from build123d import *

# Parameters (mm, degrees)
BOSS_EXTRUDE1_DEPTH = 4
SKETCH2_R           = 2.5
CUT_EXTRUDE1_DEPTH  = 4
LPATTERN1_COUNT     = 3
LPATTERN1_PITCH     = 20
SKETCH3_R           = 2.5
CUT_EXTRUDE2_DEPTH  = 4
FILLET1_R           = 0.1


with BuildPart() as part:
    # Sketch1 → Boss-Extrude1 (new body)
    with BuildSketch(Plane.XY):
        Polygon((20, 60), (40, 60), (60, 20), (60, 0), (0, 0), (0, 20), align=None)
    extrude(amount=-BOSS_EXTRUDE1_DEPTH)

    # Sketch2 → Cut-Extrude1 (cut)
    with BuildSketch(Plane.XY):
        with Locations((30, 10)):
            Circle(SKETCH2_R)
    cut_extrude1 = extrude(amount=-CUT_EXTRUDE1_DEPTH, mode=Mode.SUBTRACT)

    # LPattern1: Cut-Extrude1 ×3
    with Locations(*[(0, i * LPATTERN1_PITCH, 0) for i in range(1, LPATTERN1_COUNT)]):
        add(cut_extrude1, mode=Mode.SUBTRACT)

    # Sketch3 → Cut-Extrude2 (cut)
    with BuildSketch(Plane.XY):
        with Locations((10, 10)):
            Circle(SKETCH3_R)
        with Locations((50, 10)):
            Circle(SKETCH3_R)
    extrude(amount=-CUT_EXTRUDE2_DEPTH, mode=Mode.SUBTRACT)

    # Fillet1
    fillet1_edges = [part.edges().sort_by_distance(p)[0] for p in [
        (0, 0, -2),
        (0, 20, -2),
        (20, 60, -2),
        (40, 60, -2),
        (60, 20, -2),
        (60, 0, -2),
    ]]
    fillet(fillet1_edges, radius=FILLET1_R)


solid = part.part
Work out the finished part from the listing and answer in its coordinate system (mm). Round coordinates to 2 decimals unless told otherwise and drop trailing zeros. Write each loop counter-clockwise with the first axis right and the second up, starting at its lowest first coordinate (ties: lowest second). Pieces come first, ordered by that corner, then holes. Notation, with made-up numbers: (74.5, -8.75) -> (92.5, -8.75) arc R25 cw to (92.5, 16.25) -> close; hole circle Ø2 at (-15, 47). An arc over 180 degrees is marked (long way). Answer as CSV lines item,"result". Start each with the question number.
(1) The part is cut by section C-C, the plane x = 30. Give the vertices of the cut face in (y, z).
(2) Find the intervals of material crossed by probe 1 along Y at (x, z) = (30, -2.7); probe 2 along Y at (x, z) = (29, -1.85); probe 3 along Y at (x, z) = (10, -2.95), in increasing order.
(3) The part is cut by section A-A, the plane y = 31.5. Give the vertices of the cut face in (x, z).
(4) Each of these flat-tipped pins is pushed along its axis until it touches: pin 1 (8 mm diameter, centred on x = 15, y = 53, fed in from +Z); pin 2 (1 mm diameter, centred on y = 49.5, z = -3.5, fed in from +X). Where does it stop, or does it pass through?
(5) The mould has two halves that part along Y. Classify faces 1 (the cylindrical face through (28.16, 51.69, -1.97)), 2 (the flat face through (30, 0, -2)), 3 (the flat face through (10, 40, -2)), 4 (the flat face through (0, 10, -2)): +Y half, -Y half, draft (parallel to the pull), parting line (faces both ways), or undercut.
(6) The part is cut by section B-B, the plane z = -2.55. Give the vertices of the cut face in (x, y).
Output values:
1,outline,"(0, -4) -> (7.5, -4) -> (7.5, 0) -> (0, 0) -> close; (12.5, -4) -> (27.5, -4) -> (27.5, 0) -> (12.5, 0) -> close; (32.5, -4) -> (47.5, -4) -> (47.5, 0) -> (32.5, 0) -> close; (52.5, -4) -> (60, -4) -> (60, 0) -> (52.5, 0) -> close"
2,probe 1,"y = 0 to 7.5, 12.5 to 27.5, 32.5 to 47.5, 52.5 to 60"
2,probe 2,"y = 0 to 7.71, 12.29 to 27.71, 32.29 to 47.71, 52.29 to 60"
2,probe 3,"y = 0 to 7.5, 12.5 to 40"
3,outline,"(5.75, -4) -> (28, -4) -> (28, 0) -> (5.75, 0) -> close; (32, -4) -> (54.25, -4) -> (54.25, 0) -> (32, 0) -> close"
4,pin 1,"stops at z = 0"
4,pin 2,"stops at x = 45.5"
5,face 1,"undercut"
5,face 2,"-Y half"
5,face 3,"+Y half"
5,face 4,"draft"
6,outline,"(0, 0.1) arc R0.1 ccw to (0.1, 0) -> (59.9, 0) arc R0.1 ccw to (60, 0.1) -> (60, 19.98) arc R0.1 ccw to (59.99, 20.02) -> (40.03, 59.94) arc R0.1 ccw to (39.94, 60) -> (20.06, 60) arc R0.1 ccw to (19.97, 59.94) -> (0.01, 20.02) arc R0.1 ccw to (0, 19.98) -> close; hole circle Ø5 at (10, 10); hole circle Ø5 at (30, 10); hole circle Ø5 at (30, 30); hole circle Ø5 at (30, 50); hole circle Ø5 at (50, 10)"
